The model under review builds one solid part; all positions refer to its coordinate system, in mm. Coordinates: 2 decimals unless noted, no trailing zeros. Write each loop counter-clockwise with the first axis right and the second up, starting at its lowest first coordinate (ties: lowest second). Pieces come first, ordered by that corner, then holes. Notation, with made-up numbers: (-32, 16) - (-7, 16) arc R31 ccw to (-7, 55) - close; hole circle Ø5 at (78.5, -10.75). An arc over 180 degrees is marked (long way). Use one line per item in the form item = value. Start each with the question number.
```python
from build123d import *

# Parameters (mm, degrees)
SKETCH1_R           = 2.55
SKETCH1_R_2         = 1.5
SKETCH1_R_3         = 12.5
SKETCH1_R_4         = 2.466704156
BOSS_EXTRUDE1_DEPTH = 3


with BuildPart() as part:
    # Sketch1 → Boss-Extrude1 (new body)
    with BuildSketch(Plane(origin=(0, 0, 0), x_dir=(1, 0, 0), z_dir=(0, 1, 0))):
        with BuildLine():
            Line((57.086176903, 28.881843054), (-16.913823097, 28.881843054))
            ThreePointArc((-16.913823097, 28.881843054), (-19.742250221, 27.710270179), (-20.913823097, 24.881843054))
            Line((-20.913823097, 24.881843054), (-20.913823097, -6.618156946))
            ThreePointArc((-20.913823097, -6.618156946), (-19.742250221, -9.44658407), (-16.913823097, -10.618156946))
            Line((-16.913823097, -10.618156946), (57.086176903, -10.618156946))
            ThreePointArc((57.086176903, -10.618156946), (59.914604028, -9.44658407), (61.086176903, -6.618156946))
            Line((61.086176903, -6.618156946), (61.086176903, 24.881843054))
            ThreePointArc((61.086176903, 24.881843054), (59.914604028, 27.710270179), (57.086176903, 28.881843054))
        make_face()
        with Locations(Location((-12.713823097, -0.868156946, 0), (0, 0, 270))):
            Circle(SKETCH1_R, mode=Mode.SUBTRACT)
        with Locations(Location((7.286176903, -0.868156946, 0), (0, 0, 270))):
            Circle(SKETCH1_R, mode=Mode.SUBTRACT)
        with Locations(Location((-12.713823097, 9.131843054, 0), (0, 0, 270))):
            Circle(SKETCH1_R, mode=Mode.SUBTRACT)
        with Locations(Location((7.286176903, 9.131843054, 0), (0, 0, 270))):
            Circle(SKETCH1_R, mode=Mode.SUBTRACT)
        with BuildLine():
            Line((27.932192414, -4.964172457), (25.432192414, -7.464172457))
            ThreePointArc((25.432192414, -7.464172457), (23.240161393, -7.464172457), (23.240161393, -5.272141435))
            Line((23.240161393, -5.272141435), (25.740161393, -2.772141435))
            ThreePointArc((25.740161393, -2.772141435), (27.932192414, -2.772141435), (27.932192414, -4.964172457))
        make_face(mode=Mode.SUBTRACT)
        with BuildLine():
            Line((53.932192414, -2.772141435), (56.432192414, -5.272141435))
            ThreePointArc((56.432192414, -5.272141435), (56.432192414, -7.464172457), (54.240161393, -7.464172457))
            Line((54.240161393, -7.464172457), (51.740161393, -4.964172457))
            ThreePointArc((51.740161393, -4.964172457), (51.740161393, -2.772141435), (53.932192414, -2.772141435))
        make_face(mode=Mode.SUBTRACT)
        with Locations(Location((25.105765127, 5.791209645, 0), (0, 0, 270))):
            Circle(SKETCH1_R_2, mode=Mode.SUBTRACT)
        with Locations(Location((39.836176903, 9.131843054, 0), (0, 0, 270))):
            Circle(SKETCH1_R_3, mode=Mode.SUBTRACT)
        with Locations(Location((50.977423293, 0.467225819, 0), (0, 0, 270))):
            Circle(SKETCH1_R_2, mode=Mode.SUBTRACT)
        with Locations(Location((-12.713823097, 19.131843054, 0), (0, 0, 270))):
            Circle(SKETCH1_R_4, mode=Mode.SUBTRACT)
        with Locations(Location((7.286176903, 19.131843054, 0), (0, 0, 270))):
            Circle(SKETCH1_R, mode=Mode.SUBTRACT)
        with Locations(Location((54.051226788, 15.404234625, 0), (0, 0, 270))):
            Circle(SKETCH1_R_2, mode=Mode.SUBTRACT)
        with BuildLine():
            Line((25.740161393, 21.035827543), (23.240161393, 23.535827543))
            ThreePointArc((23.240161393, 23.535827543), (23.240161393, 25.727858565), (25.432192414, 25.727858565))
            Line((25.432192414, 25.727858565), (27.932192414, 23.227858565))
            ThreePointArc((27.932192414, 23.227858565), (28.251915532, 22.762861387), (28.383986105, 22.214224337))
            ThreePointArc((28.383986105, 22.214224337), (29.31019372, 21.713960247), (29.679568623, 20.728218451))
            ThreePointArc((29.679568623, 20.728218451), (28.24918667, 19.22983488), (26.686030853, 20.5891324))
            ThreePointArc((26.686030853, 20.5891324), (26.174275251, 20.730277429), (25.740161393, 21.035827543))
        make_face(mode=Mode.SUBTRACT)
        with BuildLine():
            ThreePointArc((54.240161393, 25.727858565), (56.432192414, 25.727858565), (56.432192414, 23.535827543))
            Line((56.432192414, 23.535827543), (53.932192414, 21.035827543))
            ThreePointArc((53.932192414, 21.035827543), (51.740161393, 21.035827543), (51.740161393, 23.227858565))
            Line((51.740161393, 23.227858565), (54.240161393, 25.727858565))
        make_face(mode=Mode.SUBTRACT)
        with Locations(Location((42.652299453, 25.534730941, 0), (0, 0, 270))):
            Circle(SKETCH1_R_2, mode=Mode.SUBTRACT)
    extrude(amount=BOSS_EXTRUDE1_DEPTH)


solid = part.part
```
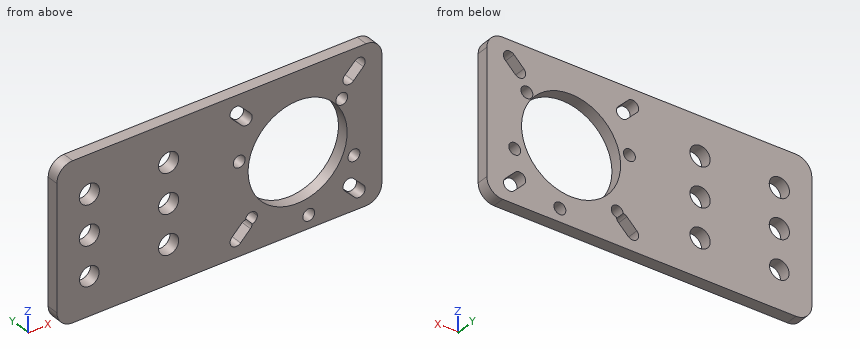
1. Take a section at C-C (z = -3.5). State the section outline as (x, y) points.
2. For L1, parallel to X at y = 2.35, z = -9; L2, parallel to X at y = 2.45, z = 7.5; L3, parallel to X at y = 2.45, z = -23.5, list the stretches that pass through material, from the lowest coordinate up.
3. Take a section at A-A (x = -13.5). State the section outline as (y, z) points.
4. Take a section at B-B (z = -9). State the section outline as (x, y) points.
5. For P1, Ø4.5, axis at x = -12.71, z = -9.13, coming from the +Y side, flat-tipped, find the tip position at first contact; note if it passes through.
6. Take a section at D-D (y = 0.9). Count the separate pieces of the cut face and the enclosed holes in it, plus the area to 3 significant figures.
Returned:
q1.outline = (-20.91, 0) - (28.68, 0) - (28.68, 3) - (-20.91, 3) - close; (51, 0) - (61.09, 0) - (61.09, 3) - (51, 3) - close
q2.L1 = -20.91 to -15.26, -10.17 to 4.74, 9.83 to 27.34, 52.34 to 61.09
q2.L2 = -20.82 to 23.28, 25.4 to 54.28, 56.4 to 60.99
q2.L3 = -20.91 to 23.28, 27.66 to 52.01, 56.4 to 61.09
q3.outline = (0, -28.88) - (3, -28.88) - (3, -21.47) - (0, -21.47) - close; (0, -16.79) - (3, -16.79) - (3, -11.56) - (0, -11.56) - close; (0, -6.71) - (3, -6.71) - (3, -1.56) - (0, -1.56) - close; (0, 3.29) - (3, 3.29) - (3, 10.62) - (0, 10.62) - close
q4.outline = (-20.91, 0) - (-15.26, 0) - (-15.26, 3) - (-20.91, 3) - close; (-10.17, 0) - (4.74, 0) - (4.74, 3) - (-10.17, 3) - close; (9.83, 0) - (27.34, 0) - (27.34, 3) - (9.83, 3) - close; (52.34, 0) - (61.09, 0) - (61.09, 3) - (52.34, 3) - close
q5.P1 = through
q6.separate_pieces = 1
q6.enclosed_holes = 15
q6.area = 2,510 mm²
